```python
from build123d import *

# Parameters (mm, degrees)
BOSS_EXTRUDE1_DEPTH                       = 3.175
F_6_CLEARANCE_HOLE1_D                     = 4.3053
CUT_EXTRUDE1_DEPTH                        = 4.175
SKETCH5_R                                 = 6.35
SKETCH5_R_2                               = 1.651
CUT_EXTRUDE2_DEPTH                        = 4.175
F_1_4_CLEARANCE_HOLE1_D                   = 7.14248
BOSS_EXTRUDE2_DEPTH                       = 3.175
CUT_EXTRUDE3_DEPTH                        = 0.635
CSK_FOR_6_FLAT_HEAD_MACHINE_SCREW_2_COUNT = 2
CSK_FOR_6_FLAT_HEAD_MACHINE_SCREW_2_PITCH = 28.321
CSK_FOR_6_FLAT_HEAD_MACHINE_SCREW_3_COUNT = 2
CSK_FOR_6_FLAT_HEAD_MACHINE_SCREW_3_PITCH = 23.555999878


with BuildPart() as part:
    # Sketch1 → Boss-Extrude1 (new body)
    with BuildSketch(Plane.XY):
        Polygon((-65.0875, 0), (-65.0875, -88.9), (-17.4625, -88.9), (0, -71.4375), (0, 0), align=None)
    extrude(amount=-BOSS_EXTRUDE1_DEPTH)

    # #6 Clearance Hole1 (through all)
    with Locations(Plane.XY):
        with Locations((-58.7375, -6.35), (-6.35, -6.35), (-23.1775, -12.7), (-57.15, -67.31), (-58.7375, -82.55)):
            Hole(F_6_CLEARANCE_HOLE1_D / 2)

    # Sketch4 → Cut-Extrude1 (cut, through all)
    with BuildSketch(Plane.XY):
        with BuildLine():
            Line((-49.3395, -50.8), (-49.3395, -43.4529836))
            ThreePointArc((-49.3395, -43.4529836), (-46.0375, -13.335), (-42.7355, -43.4529836))
            Line((-42.7355, -43.4529836), (-42.7355, -50.8))
            ThreePointArc((-42.7355, -50.8), (-46.0375, -54.102), (-49.3395, -50.8))
        make_face()
    extrude(amount=-CUT_EXTRUDE1_DEPTH, mode=Mode.SUBTRACT)

    # Sketch5 → Cut-Extrude2 (cut, through all)
    with BuildSketch(Plane.XY):
        with Locations((-16.8275, -27.94)):
            Circle(SKETCH5_R)
        with Locations((-16.8275, -18.9484)):
            Circle(SKETCH5_R_2)
    extrude(amount=-CUT_EXTRUDE2_DEPTH, mode=Mode.SUBTRACT)

    # 1/4 Clearance Hole1 (through all)
    with Locations(Plane.XY):
        with Locations((-9.2075, -65.0875)):
            Hole(F_1_4_CLEARANCE_HOLE1_D / 2)

    # Sketch8 → Boss-Extrude2 (add, through all)
    with BuildSketch(Plane(origin=(0, 0, -3.175), x_dir=(-1, 0, 0), z_dir=(0, 0, -1))):
        with BuildLine():
            Line((52.1335, -39.716309797), (52.1335, -42.542690718))
            ThreePointArc((52.1335, -42.542690718), (46.0375, -13.335), (39.9415, -42.542690718))
            Line((39.9415, -42.542690718), (39.9415, -39.716309797))
            ThreePointArc((39.9415, -39.716309797), (38.993964439, -39.142809934), (38.1, -38.488934323))
            Line((38.1, -38.488934323), (38.1, -28.575))
            ThreePointArc((38.1, -28.575), (46.0375, -20.6375), (53.975, -28.575))
            Line((53.975, -28.575), (53.975, -38.488934323))
            ThreePointArc((53.975, -38.488934323), (53.081035561, -39.142809934), (52.1335, -39.716309797))
        make_face()
    extrude(amount=-BOSS_EXTRUDE2_DEPTH)

    # Sketch9 → Cut-Extrude3 (cut)
    with BuildSketch(Plane.XY):
        with BuildLine():
            Line((-52.1335, -39.716309797), (-52.1335, -42.542690718))
            ThreePointArc((-52.1335, -42.542690718), (-46.0375, -13.335), (-39.9415, -42.542690718))
            Line((-39.9415, -42.542690718), (-39.9415, -39.716309797))
            ThreePointArc((-39.9415, -39.716309797), (-38.993964439, -39.142809934), (-38.1, -38.488934323))
            ThreePointArc((-38.1, -38.488934323), (-46.0375, -15.875), (-53.975, -38.488934323))
            ThreePointArc((-53.975, -38.488934323), (-53.081035561, -39.142809934), (-52.1335, -39.716309797))
        make_face()
    extrude(amount=-CUT_EXTRUDE3_DEPTH, mode=Mode.SUBTRACT)

    # Sketch10 → CSK for #6 Flat Head Machine Screw (100)1 (revolve, cut)
    with BuildSketch(Plane(origin=(-31.877, -53.091877173, 0), x_dir=(0, -1, 0), z_dir=(1, 0, 0))):
        Polygon((0, 0), (0, 3.175), (2.15265, 3.175), (2.15265, 1.420893136), (3.8460045, 0), align=None)
    csk_for_6_flat_head_machine_screw_100 = revolve(axis=Axis((-31.877, -53.091877173, 6.35), (0, 0, -1)), mode=Mode.SUBTRACT)

    # CSK for _6 Flat Head Machine Screw _ 2: CSK for #6 Flat Head Machine Screw (100)1 ×2
    with Locations(*[(-i * CSK_FOR_6_FLAT_HEAD_MACHINE_SCREW_2_PITCH, 0, 0) for i in range(1, CSK_FOR_6_FLAT_HEAD_MACHINE_SCREW_2_COUNT)]):
        add(csk_for_6_flat_head_machine_screw_100, mode=Mode.SUBTRACT)

    # CSK for _6 Flat Head Machine Screw _ 3: CSK for #6 Flat Head Machine Screw (100)1 ×2
    with Locations(*[(i * CSK_FOR_6_FLAT_HEAD_MACHINE_SCREW_3_PITCH, 0, 0) for i in range(1, CSK_FOR_6_FLAT_HEAD_MACHINE_SCREW_3_COUNT)]):
        add(csk_for_6_flat_head_machine_screw_100, mode=Mode.SUBTRACT)


solid = part.part
```
Verification items for the finished model (mm, model axes). A direction names the side the tool comes from. Give positions to 0.01 mm unless a question says otherwise; leave off trailing zeros. Order: outer loops, then holes, each group sorted by start corner. A loop starts at its lowest first (then second) coordinate and runs counter-clockwise, first axis right, second up. Notation, with made-up numbers: M -7.5,62 L 14.5,62 A15 cw 14.5,90 Z; hole C -38.75,86 d3. An arc over 180 degrees is marked long. Answer in a Markdown table with one row per item. Add a question column.
Item 1: Scan lines: probe 1 along X at (y, z) = (-23, -0.05); probe 2 along Y at (x, z) = (-59.5, -1.95); probe 3 along Y at (x, z) = (-57.15, -1.5). Record each from-to range of solid material in increasing order. Write a range as from..to.
Item 2: Section check A-A, the plane y = -6.35. Enter the section's corners in (x, z) (1 decimal), and give its area (3 significant figures).
Item 3: Tool access check on faces 1 (the flat face through (-42, -88.9, -2)), 2 (the flat face through (-40, -17, -0.635)), 3 (the cylindrical face through (-46, -54.1, -1.6)). Record the directions out of +Z, -Z, +X, -X, +Y, -Y that give a thin tool (end or side, any length) a straight path to the whole face; none if there is none.
Item 4: Section check B-B, the plane x = -41. Enter the section's corners in (y, z) (3 decimals).
Item 5: Mould release check, pull along Y, two halves, no side actions. Record for faces 4 (the cylindrical face through (-57.151, -81.095, -1.61)), 5 (the flat face through (-32, 0, -2)), 6 (the flat face through (-38.1, -34, -2)), 7 (the flat face through (-8.85, -80.29, -1.57)): released by +Y, released by -Y, zero draft, split by the parting line, or undercut.
Item 6: Section check C-C, the plane z = -2.6. State how many separate pieces and enclosed holes the cut face has, and give its area (3 significant figures).
Filled sheet:
| question | item | result |
|---|---|---|
| 1 | probe 1 | x = -65.09..-60.22, -57.45..-51.69, -40.39..-34.63, -31.85..-20.82, -12.84..0 |
| 1 | probe 2 | y = -88.9..-84.56, -80.54..-55.13, -51.06..-8.36, -4.34..0 |
| 1 | probe 3 | y = -88.9..-84, -81.1..-69.46, -65.16..-7.8, -4.9..0 |
| 2 | outline | M -65.1,-3.2 L -60.9,-3.2 L -60.9,0 L -65.1,0 Z; M -56.6,-3.2 L -8.5,-3.2 L -8.5,0 L -56.6,0 Z; M -4.2,-3.2 L 0,-3.2 L 0,0 L -4.2,0 Z |
| 2 | area | 179 mm^2 |
| 3 | face 1 | +Z, -Z, +X, -X, -Y |
| 3 | face 2 | +Z |
| 3 | face 3 | +Z, -Z |
| 4 | outline | M -88.9,-3.175 L -42.958,-3.175 L -42.958,0 L -88.9,0 Z; M -22.441,-3.175 L 0,-3.175 L 0,0 L -14.192,0 L -14.192,-0.635 L -16.917,-0.635 L -16.917,0 L -22.441,0 Z |
| 5 | face 4 | undercut |
| 5 | face 5 | released by +Y |
| 5 | face 6 | undercut |
| 5 | face 7 | released by -Y |
| 6 | separate pieces | 1 |
| 6 | enclosed holes | 12 |
| 6 | area | 4,960 mm^2 |
